Geometry check sheet. Reference: the model listing, model coordinates, mm. Face numbers are marked on the shaded views. Give positions to 0.01 mm unless a question says otherwise; leave off trailing zeros. Order: outer loops, then holes, each group sorted by start corner. A loop starts at its lowest first (then second) coordinate and runs counter-clockwise, first axis right, second up. Notation, with made-up numbers: M 87,22 L 139,22 A12 ccw 139,31 Z; hole C 69,78 d3. An arc over 180 degrees is marked long. Put each result on its own line as item: value. Start each with the question number.
Q1. Go/stop test with flat-tipped pins: pin 1 (1.5 mm diameter, centred on y = -4.5, z = -25.5, fed in from -X); pin 2 (1 mm diameter, centred on y = -17.5, z = -9.5, fed in from +X); pin 3 (4 mm diameter, centred on x = -15.5, y = -7.5, fed in from -Z). Record where each tip stops, or that it passes through.
Q2. Section check A-A on x = -18.5. Record the cut outline in (y, z), then the cut area to 3 significant figures.
Q3. Section check B-B on z = 0. Record the cut outline in (x, y), then the cut area to 3 significant figures.
Q4. Material ranges on L1, parallel to X at y = -14.5, z = 0; L2, parallel to Y at x = -31.5, z = 7.5; L3, parallel to Y at x = -35, z = -7.5, recorded low to high.
Q5. Section check D-D on z = 18. Record the cut outline in (x, y).
Q6. Section check C-C on y = -14.5. Record the cut outline in (x, z), then the cut area to 3 significant figures.
Q7. Mould release check, pull along Z, two halves, no side actions. Record for the marked faces 1, 2 and 3: +Z half, -Z half, draft (parallel to the pull), parting line (faces both ways), or undercut.
```python
from build123d import *

# Parameters (mm, degrees)
SKETCH4_R               = 1.5
BOSS_EXTRUDE1_DEPTH     = 5
SKETCH5_W               = 25
SKETCH5_H               = 6.621086299
CUT_EXTRUDE5_DEPTH      = 5
FILLET1_R               = 1
CUT_EXTRUDE9_DEPTH      = 77.752708656
CUT_EXTRUDE9_DEPTH_BACK = 15
MOVE_FACE1_BY           = 0.1


with BuildPart() as part:
    # Sketch2 → Revolve3 (revolve)
    with BuildSketch(Plane.XY, mode=Mode.PRIVATE) as revolve3_sk:
        Polygon((1.5, -20), (1.5, -5), (11.5, -5), (11.5, -3.1), (-18.5, -3.1), (-18.5, -5.1), (-2.5, -5.1), (-2.5, -20), align=None)
    revolve(revolve3_sk.sketch.rotate(Axis((-18.5, -3.1, 0), (0, -1, 0)), 90), axis=Axis((-18.5, -3.1, 0), (0, -1, 0)))

    # Sketch4 → Boss-Extrude1 (add)
    with BuildSketch(Plane.XZ.offset(20)):
        with Locations(Location((-2.911542732, -9, 0), (0, 0, 90))):
            Circle(SKETCH4_R)
        with Locations(Location((-18.5, 18, 0), (0, 0, 90))):
            Circle(SKETCH4_R)
        with Locations(Location((-34.088457268, -9, 0), (0, 0, 90))):
            Circle(SKETCH4_R)
    extrude(amount=BOSS_EXTRUDE1_DEPTH)

    # Sketch5 → Cut-Extrude5 (cut)
    with BuildSketch(Plane(origin=(0, -3.1, 0), x_dir=(1, 0, 0), z_dir=(0, 1, 0))):
        with Locations((-18.475404108, 27.289504664)):
            Rectangle(SKETCH5_W, SKETCH5_H)
    extrude(amount=-CUT_EXTRUDE5_DEPTH, mode=Mode.SUBTRACT)

    # Fillet1
    fillet1_edges = [part.edges().sort_by_distance(p)[0] for p in [
        (-5.975404108, -4.05, -23.978961514),
        (-30.975404108, -4.05, -23.978961514),
    ]]
    fillet(fillet1_edges, radius=FILLET1_R)

    # Sketch6 → Cut-Extrude9 (cut, two sides)
    with BuildSketch(Plane(origin=(0, 0, -23.978961514), x_dir=(-1, 0, 0), z_dir=(0, 0, -1))) as cut_extrude9_sk:
        Polygon((18.487702054, -11.55), (18.478169327, -5), (9.487702054, -5), (9.487702054, -11.55), align=None)
        Polygon((27.487702054, -5), (18.478169327, -5), (18.487702054, -11.55), (27.487702054, -11.55), align=None)
    extrude(amount=CUT_EXTRUDE9_DEPTH, mode=Mode.SUBTRACT)
    extrude(cut_extrude9_sk.sketch, amount=-CUT_EXTRUDE9_DEPTH_BACK, mode=Mode.SUBTRACT)

    # Move Face1: a face moved inward by 0.1
    extrude(part.faces().sort_by_distance((-18.501355787, -5.1, 1.924560303))[0], amount=MOVE_FACE1_BY, dir=(0, 1, 0), mode=Mode.SUBTRACT)


solid = part.part
```
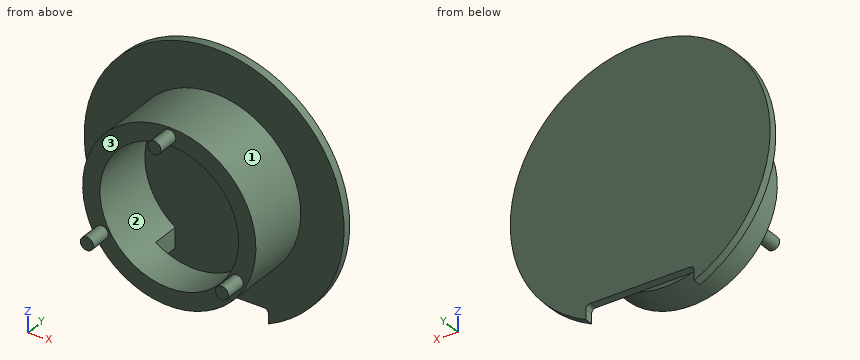
Results found:
1. pin 1: stops at x = -35.45
1. pin 2: stops at x = -0.64
1. pin 3: stops at z = 15.2
2. outline: M -25,16.5 L -20,16.5 L -20,16 L -5,16 L -5,-23.98 L -3.1,-23.98 L -3.1,30 L -5,30 L -5,20 L -20,20 L -20,19.5 L -25,19.5 Z; M -20,-20 L -11.55,-20 L -11.55,-16 L -20,-16 Z
2. area: 211 mm^2
3. outline: M -48.5,-5 L -38.5,-5 L -38.5,-20 L -34.5,-20 L -34.5,-5 L -2.5,-5 L -2.5,-20 L 1.5,-20 L 1.5,-5 L 11.5,-5 L 11.5,-3.1 L -48.5,-3.1 Z
3. area: 234 mm^2
4. L1: x = -38.5 to -34.5, -2.5 to 1.5
4. L2: y = -5 to -3.1
4. L3: y = -20 to -3.1
5. outline: M -42.5,-5 L -27.22,-5 L -27.22,-20 L -20,-20 L -20,-25 L -17,-25 L -17,-20 L -9.78,-20 L -9.78,-5 L 5.5,-5 L 5.5,-3.1 L -42.5,-3.1 Z
6. outline: C -18.5,0 d40; hole C -18.5,0 d32
6. area: 452 mm^2
7. face 1: parting line
7. face 2: undercut
7. face 3: draft
